Here's the drawing with two shaded views (mm, measured from the low corner). I have some questions. Give positions to 0.01 mm unless a question says otherwise; leave off trailing zeros. Write each loop counter-clockwise with the first axis right and the second up, starting at its lowest first coordinate (ties: lowest second). Pieces come first, ordered by that corner, then holes.
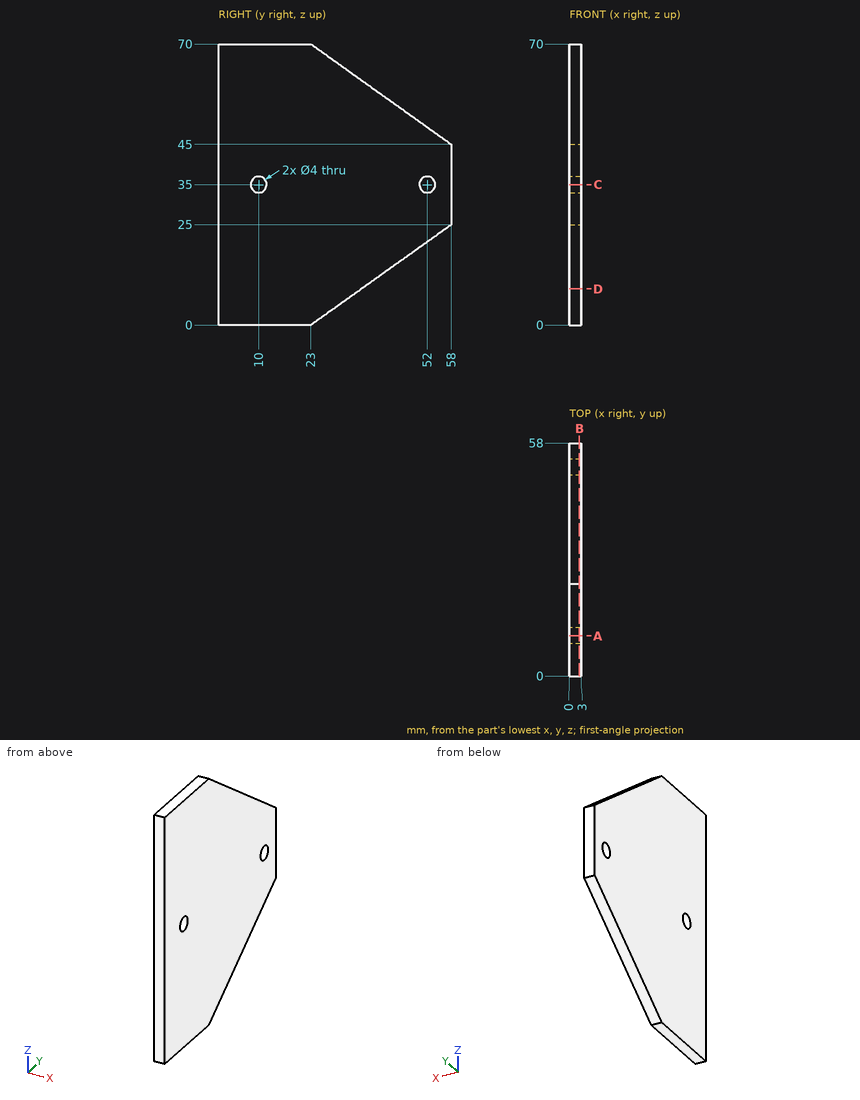
(1) Imagine slicing it at B-B, the plane x = 2.45. Write out the boundary of the cut face in (y, z).
Returned:
outline: (0, 0) - (23, 0) - (58, 25) - (58, 45) - (23, 70) - (0, 70) - close; hole circle Ø4 at (10, 35); hole circle Ø4 at (52, 35)
(2) Imagine slicing it at A-A, the plane y = 10. Write out the boundary of the cut face in (x, z), plus the area to 3 significant figures.
Returned:
outline: (0, 0) - (3, 0) - (3, 33) - (0, 33) - close; (0, 37) - (3, 37) - (3, 70) - (0, 70) - close
area: 198 mm2
(3) If I drill on L1, parallel to Y at x = 1.85, z = 35; L2, parallel to Z at x = 0.95, y = 50.5; L3, parallel to Z at x = 1.7, y = 24.5, over which ranges is the centre line in solid material (lowest first)?
Returned:
L1: y = 0 to 8, 12 to 50, 54 to 58
L2: z = 19.64 to 33.68, 36.32 to 50.36
L3: z = 1.07 to 68.93
(4) Imagine slicing it at D-D, the plane z = 9. Write out the boundary of the cut face in (x, y), plus the area to 3 significant figures.
Returned:
outline: (0, 0) - (3, 0) - (3, 35.6) - (0, 35.6) - close
area: 107 mm2
(5) Will this pin go through, and if not, where does the flat tip stop? P1, Ø2.5, axis at y = 10, z = 35, coming from the +X side.
Returned:
P1: passes through
(6) Imagine slicing it at C-C, the plane z = 35. Write out the boundary of the cut face in (x, y).
Returned:
outline: (0, 0) - (3, 0) - (3, 8) - (0, 8) - close; (0, 12) - (3, 12) - (3, 50) - (0, 50) - close; (0, 54) - (3, 54) - (3, 58) - (0, 58) - close
